from build123d import *

# Parameters (mm, degrees)
F0_W     = 533.4
F0_H     = 863.6
F1_DEPTH = 12.7
F3_DEPTH = 12.701
F4_R     = 38.1


with BuildPart() as f1:
    # F0 (on Front) → F1 (new body)
    with BuildSketch(Plane.XZ):
        Rectangle(F0_W, F0_H)
    extrude(amount=F1_DEPTH)

    # F2 (on face) → F3 (cut, through all)
    with BuildSketch(Plane.XZ.offset(12.7)):
        with BuildLine():
            Line((-61.394244, -355.6), (-266.7, 0))
            Line((-266.7, 0), (-266.7, -431.8))
            Line((-266.7, -431.8), (-105.388335, -431.8))
            ThreePointArc((-105.388335, -431.8), (-61.394244, -406.4), (-61.394244, -355.6))
        make_face()
        Polygon((-105.388335, 25.4), (158.576208, -431.8), (266.7, -431.8), (266.7, 25.4), align=None)
    extrude(amount=-F3_DEPTH, mode=Mode.SUBTRACT)

    # F4
    f4_edges = [f1.edges().sort_by_distance(p)[0] for p in [
        (-266.7, -6.35, 431.8),
        (-105.388335, -6.35, 25.4),
    ]]
    fillet(f4_edges, radius=F4_R)


solid = f1.part
Geometry check sheet. Reference: the model listing, model coordinates, mm. A direction names the side the tool comes from. Round coordinates to 2 decimals unless told otherwise and drop trailing zeros. Write each loop counter-clockwise with the first axis right and the second up, starting at its lowest first coordinate (ties: lowest second). Pieces come first, ordered by that corner, then holes. Notation, with made-up numbers: (-36.75, 18) -> (-28.75, 18) arc R5 ccw to (-28.75, 26) -> close; hole circle Ø1 at (60, 71.5). An arc over 180 degrees is marked (long way). One line per item, written item: value. Start each with the question number.
(1) Scan lines: line 1 (Z direction, x = -73.5, y = -8.5); line 2 (Z direction, x = 84.5, y = -1.25); line 3 (Z direction, x = -24.5, y = -7). Record each from-to range of solid material in increasing order. Write a range as [from, to].
(2) Cross-section at A-A, the plane x = 107. Record the cut outline in (y, z), and give its area (3 significant figures).
(3) Go/stop test with flat-tipped pins: pin 1 Ø1 at (y, z) = (-9, -6.5) entering from -X; pin 2 Ø1 at (y, z) = (-4, -272) entering from +X. Record where each tip stops, or that it passes through.
(4) Cross-section at C-C, the plane x = 214.5. Record the cut outline in (y, z).
(5) Cross-section at D-D, the plane z = -243.5. Record the cut outline in (x, y).
(6) Access from +Z, -Z, +X, -X, +Y, -Y to the whole of each face (thin tool, end or side, straight path). Record for faces 1 (the flat face through (-162.61, -6.44, -180.29)), 2 (the flat face through (41.47, -6.44, -228.97)), 3 (the flat face through (-4, -12.7, 102)).
(7) Draft check along Z on faces 4 (the cylindrical face through (-255.84, -6.44, 420.34)), 5 (the flat face through (-4, 0, 102)), 6 (the cylindrical face through (-72.11, -6.26, 6.83)). Enter one of: +Z half, -Z half, draft (parallel to the pull), parting line (faces both ways), or undercut.
(8) Cross-section at B-B, the plane y = -3.5. Record the cut outline in (x, z), and give its area (3 significant figures).
Answer:
1. line 1: [-431.8, -420.54], [-334.63, -29.69], [4.29, 431.8]
1. line 2: [-431.8, -303.5], [25.4, 431.8]
1. line 3: [-431.8, -114.7], [25.4, 431.8]
2. outline: (-12.7, -431.8) -> (0, -431.8) -> (0, -342.47) -> (-12.7, -342.47) -> close; (-12.7, 25.4) -> (0, 25.4) -> (0, 431.8) -> (-12.7, 431.8) -> close
2. area: 6,300 mm²
3. pin 1: x = -263.24
3. pin 2: x = 66.6
4. outline: (-12.7, 25.4) -> (0, 25.4) -> (0, 431.8) -> (-12.7, 431.8) -> close
5. outline: (-126.12, -12.7) -> (49.86, -12.7) -> (49.86, 0) -> (-126.12, 0) -> close
6. face 1: -X, +Y, -Y
6. face 2: +X, +Y, -Y
6. face 3: +Z, -Z, +X, -X, -Y
7. face 4: +Z half
7. face 5: draft
7. face 6: undercut
8. outline: (-266.7, 0) -> (-61.39, -355.6) arc R50.8 cw to (-105.39, -431.8) -> (158.58, -431.8) -> (-72.39, -31.75) arc R38.1 cw to (-39.4, 25.4) -> (266.7, 25.4) -> (266.7, 431.8) -> (-228.6, 431.8) arc R38.1 ccw to (-266.7, 393.7) -> close
8. area: 299,000 mm²
